Could you check a few things on this model? Use its own coordinates, in mm. Face numbers are marked on the shaded views. A direction names the side the tool comes from. Round coordinates to 2 decimals unless told otherwise and drop trailing zeros. Order: outer loops, then holes, each group sorted by start corner. A loop starts at its lowest first (then second) coordinate and runs counter-clockwise, first axis right, second up.
```python
from build123d import *

# Parameters (mm, degrees)
SKETCH1_R           = 17.5
BOSS_EXTRUDE1_DEPTH = 10
SKETCH2_R           = 32.5
BOSS_EXTRUDE2_DEPTH = 5
SKETCH3_R           = 2.95
CUT_EXTRUDE1_DEPTH  = 7


with BuildPart() as part:
    # Sketch1 → Boss-Extrude1 (new body)
    with BuildSketch(Plane(origin=(0, 0, 0), x_dir=(1, 0, 0), z_dir=(0, 1, 0))):
        Circle(SKETCH1_R)
    extrude(amount=BOSS_EXTRUDE1_DEPTH)

    # Sketch2 → Boss-Extrude2 (add)
    with BuildSketch(Plane(origin=(0, 10, 0), x_dir=(1, 0, 0), z_dir=(0, 1, 0))):
        Circle(SKETCH2_R)
    extrude(amount=BOSS_EXTRUDE2_DEPTH)

    # Sketch3 → Cut-Extrude1 (cut)
    with BuildSketch(Plane(origin=(0, 15, 0), x_dir=(1, 0, 0), z_dir=(0, 1, 0))):
        with Locations((0, 25)):
            Circle(SKETCH3_R)
        with Locations((23.776412907, 7.725424859)):
            Circle(SKETCH3_R)
        with Locations((14.694631307, -20.225424859)):
            Circle(SKETCH3_R)
        with Locations((-14.694631307, -20.225424859)):
            Circle(SKETCH3_R)
        with Locations((-23.776412907, 7.725424859)):
            Circle(SKETCH3_R)
    extrude(amount=-CUT_EXTRUDE1_DEPTH, mode=Mode.SUBTRACT)


solid = part.part
```
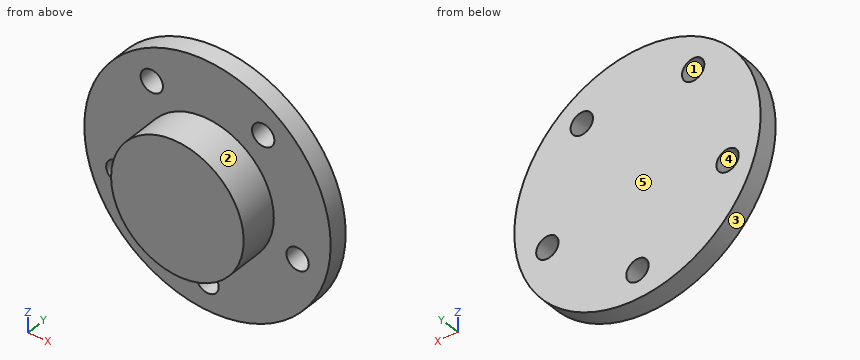
Q1. Imagine slicing it at B-B, the plane z = 0. Please give me the cut outline in (x, y), then the cut area to 3 significant figures.
Q2. I need wall thicknesses on L1, parallel to Z at x = 0, y = 12.3; L2, parallel to Y at x = 19.5, z = -14; L3, parallel to X at y = 12, z = -23. Which ranges of each line are inside material? Lowest first, please.
Q3. For P1, Ø5, axis at y = 2.5, z = -13, coming from the -X side; P2, Ø7, axis at x = -14.69, z = 20.23, coming from the -Y side; P3, Ø3, axis at x = -14.5, y = 9.5, coming from the +Z side, each with a flat end and sliding along its axis, tell me the tip position at first contact or that it passes through.
Q4. For the marked faces 1 and 2, which set-ups out of +Z, -Z, +X, -X, +Y, -Y let a thin tool reach every point of the face, with its end or its side?
Q5. Imagine slicing it at C-C, the plane z = -25. Please give me the cut outline in (x, y), then the cut area to 3 significant figures.
Q6. We'd pull the mould along X, two halves only. Please class the marked faces 3, 4 and 5: released by +X, released by -X, zero draft, split by the parting line, or undercut.
Q7. Imagine slicing it at A-A, the plane x = -24. Please give me the cut outline in (y, z), then the cut area to 3 significant figures.
Q8. Imagine slicing it at D-D, the plane y = 11. Please give me the cut outline in (x, z).
Filled in:
1. outline: (-32.5, 10) - (-17.5, 10) - (-17.5, 0) - (17.5, 0) - (17.5, 10) - (32.5, 10) - (32.5, 15) - (-32.5, 15) - close
1. area: 675 mm2
2. L1: z = -32.5 to -27.95, -22.05 to 32.5
2. L2: y = 10 to 15
2. L3: x = -22.96 to -2.17, 2.17 to 22.96
3. P1: stops at x = -14
3. P2: stops at y = 10
3. P3: stops at z = 29.75
4. face 1: +Y, -Y
4. face 2: -Y
5. outline: (-20.77, 10) - (-2.95, 10) - (-2.95, 15) - (-20.77, 15) - close; (2.95, 10) - (20.77, 10) - (20.77, 15) - (2.95, 15) - close
5. area: 178 mm2
6. face 3: split by the parting line
6. face 4: undercut
6. face 5: zero draft
7. outline: (10, -21.91) - (15, -21.91) - (15, -10.67) - (10, -10.67) - close; (10, -4.78) - (15, -4.78) - (15, 21.91) - (10, 21.91) - close
7. area: 190 mm2
8. outline: circle Ø65 at (0, 0); hole circle Ø5.9 at (-23.78, -7.73); hole circle Ø5.9 at (-14.69, 20.23); hole circle Ø5.9 at (0, -25); hole circle Ø5.9 at (14.69, 20.23); hole circle Ø5.9 at (23.78, -7.73)
